Check sheet for the modelled part. Datum: model origin and axes. Units: mm. A direction names the side the tool comes from. Give positions to 0.01 mm unless a question says otherwise; leave off trailing zeros. Order: outer loops, then holes, each group sorted by start corner. A loop starts at its lowest first (then second) coordinate and runs counter-clockwise, first axis right, second up. Notation, with made-up numbers: (-25, -34) -> (5, -34) arc R27 ccw to (5, -18) -> close; hole circle Ø2 at (26, -8.75). An arc over 180 degrees is marked (long way). Answer in a Markdown table with one row per item. Add a question column.
(1) Go/stop test with flat-tipped pins: pin 1 (8 mm diameter, centred on x = -192, y = -95.5, fed in from -Z); pin 2 (3 mm diameter, centred on y = -114, z = 4.5, fed in from +X); pin 3 (1.8 mm diameter, centred on x = -205.5, z = 2, fed in from -Y). Record where each tip stops, or that it passes through.
(2) Cross-section at A-A (x = -195). Record the cut outline in (y, z), then the cut area to 3 significant figures.
(3) Cross-section at D-D (x = -205). Record the cut outline in (y, z), then the cut area to 3 significant figures.
(4) Set-up check for faces 1 (the face through (-202.684, -113, 3)), 2 (the face through (-182.684, -71, 3)), 3 (the face through (-207, -77.263, 3)), 4 (the face through (-179, -107.263, 3)), 5 (the face through (-193, -99.191, 3)): record each of +Z, -Z, +X, -X, +Y, -Y from which the full face is reachable in a straight line by a thin tool's end or side.
(5) Release check for a two-part mould opening along X. For faces 6 (the face through (-179, -77.263, 3)), 7 (the face through (-182.684, -113, 3)), 8 (the face through (-193, -85.335, 3)) record: released by +X, released by -X, zero draft, split by the parting line, or undercut.
(6) Thickness scan on L1, parallel to Y at x = -190.5, z = 4.3; L2, parallel to Y at x = -209, z = 1.4; L3, parallel to X at y = -94, z = 5.75. Record the ranges inside material, lowest first. Write a range as [from, to].
(7) Cross-section at C-C (z = 1.3). Record the cut outline in (x, y), then the cut area to 3 significant figures.
(8) Cross-section at B-B (y = -97). Record the cut outline in (x, z), then the cut area to 3 significant figures.
```python
from build123d import *

# Parameters (mm, degrees)
BOSS_EXTRUDE1_DEPTH = 6


with BuildPart() as part:
    # Sketch1 → Boss-Extrude1 (new body)
    with BuildSketch(Plane.XY):
        Polygon((-211.428617248, -77.262954902), (-211.428617248, -107.262954902), (-202.683627049, -107.262954902), (-202.683627049, -113.262954902), (-202.683627049, -119.262954902), (-182.683627049, -119.262954902), (-182.683627049, -113.262954902), (-182.683627049, -107.262954902), (-174.549373808, -107.262954902), (-174.549373808, -77.262954902), (-182.683627049, -77.262954902), (-182.683627049, -71.262954902), (-182.683627049, -65.262954902), (-202.683627049, -65.262954902), (-202.683627049, -71.262954902), (-202.683627049, -77.262954902), align=None)
        Polygon((-184.988995528, -92.262954902), (-188.988995528, -85.334751672), (-196.988995528, -85.334751672), (-200.988995528, -92.262954902), (-196.988995528, -99.191158133), (-188.988995528, -99.191158133), align=None, mode=Mode.SUBTRACT)
    extrude(amount=BOSS_EXTRUDE1_DEPTH)


solid = part.part
```
Answer below:
| question | item | result |
|---|---|---|
| 1 | pin 1 | stops at z = 0 |
| 1 | pin 2 | stops at x = -182.68 |
| 1 | pin 3 | stops at y = -107.26 |
| 2 | outline | (-119.26, 0) -> (-99.19, 0) -> (-99.19, 6) -> (-119.26, 6) -> close; (-85.33, 0) -> (-65.26, 0) -> (-65.26, 6) -> (-85.33, 6) -> close |
| 2 | area | 241 mm² |
| 3 | outline | (-107.26, 0) -> (-77.26, 0) -> (-77.26, 6) -> (-107.26, 6) -> close |
| 3 | area | 180 mm² |
| 4 | face 1 | +Z, -Z, -X, -Y |
| 4 | face 2 | +Z, -Z, +X, +Y |
| 4 | face 3 | +Z, -Z, -X, +Y |
| 4 | face 4 | +Z, -Z, +X, -Y |
| 4 | face 5 | +Z, -Z |
| 5 | face 6 | zero draft |
| 5 | face 7 | released by +X |
| 5 | face 8 | undercut |
| 6 | L1 | y = [-119.26, -99.19], [-85.33, -65.26] |
| 6 | L2 | y = [-107.26, -77.26] |
| 6 | L3 | x = [-211.43, -199.99], [-185.99, -174.55] |
| 7 | outline | (-211.43, -107.26) -> (-202.68, -107.26) -> (-202.68, -119.26) -> (-182.68, -119.26) -> (-182.68, -107.26) -> (-174.55, -107.26) -> (-174.55, -77.26) -> (-182.68, -77.26) -> (-182.68, -65.26) -> (-202.68, -65.26) -> (-202.68, -77.26) -> (-211.43, -77.26) -> close; hole (-200.99, -92.26) -> (-196.99, -99.19) -> (-188.99, -99.19) -> (-184.99, -92.26) -> (-188.99, -85.33) -> (-196.99, -85.33) -> close |
| 7 | area | 1,420 mm² |
| 8 | outline | (-211.43, 0) -> (-198.25, 0) -> (-198.25, 6) -> (-211.43, 6) -> close; (-187.72, 0) -> (-174.55, 0) -> (-174.55, 6) -> (-187.72, 6) -> close |
| 8 | area | 158 mm² |
